Could you check a few things on this drawing? It's one solid part, dimensions in mm from its lowest x, y, z. A direction names the side the tool comes from. Give positions to 0.01 mm unless a question says otherwise; leave off trailing zeros. Write each loop counter-clockwise with the first axis right and the second up, starting at its lowest first coordinate (ties: lowest second). Pieces come first, ordered by that corner, then holes. Notation, with made-up numbers: M -14,18.25 L -10,18.25 A33 cw -10,51.25 Z; hole C 51,-26.5 d2. An arc over 180 degrees is marked long. Answer as CSV lines item,"result". Start each with the question number.
Q1. Suppose I cut it at B-B (y = 7.5). Write out the boundary of the cut face in (x, z), then the cut area to 3 significant figures.
Q2. Suppose I cut it at A-A (x = 23.5). Write out the boundary of the cut face in (y, z).
Q3. On a 3-axis mill with a long thin cutter (end or side, diameter ignored), from which of +Z, -Z, +X, -X, +Y, -Y can I reach the whole of each face in a straight line? I mean the marked faces 1 and 2. Say none if no direction works.
Q4. If I drill on line 1 along Y through (x, z) = (23.8, 37.5); line 2 along X through (y, z) = (5, 83); line 3 along Y through (x, z) = (16.25, 58.5), over which ranges is the centre line in solid material (lowest first)?
Q5. Suppose I cut it at C-C (z = 37.5). Write out the boundary of the cut face in (x, y).
Q6. Suppose I cut it at D-D (z = 55.5). Write out the boundary of the cut face in (x, y), then the cut area to 3 significant figures.
Q7. For pin 1 (2 mm diameter, centred on x = 8.5, z = 69.5, fed in from +Y); pin 2 (3 mm diameter, centred on y = 9, z = 34, fed in from -X), each with a flat end and sliding along its axis, tell me the tip position at first contact or that it passes through.
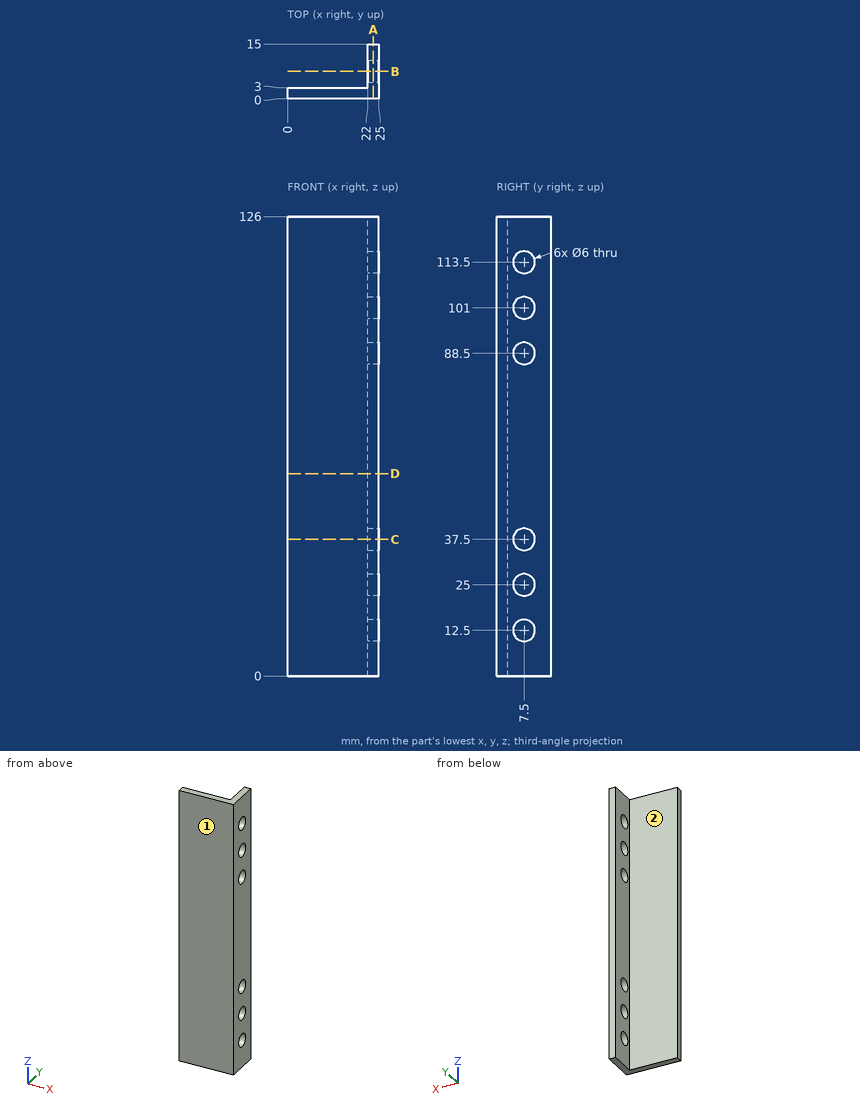
Resolved:
1,outline,"M 22,0 L 25,0 L 25,9.5 L 22,9.5 Z; M 22,15.5 L 25,15.5 L 25,22 L 22,22 Z; M 22,28 L 25,28 L 25,34.5 L 22,34.5 Z; M 22,40.5 L 25,40.5 L 25,85.5 L 22,85.5 Z; M 22,91.5 L 25,91.5 L 25,98 L 22,98 Z; M 22,104 L 25,104 L 25,110.5 L 22,110.5 Z; M 22,116.5 L 25,116.5 L 25,126 L 22,126 Z"
1,area,"270 mm^2"
2,outline,"M 0,0 L 15,0 L 15,126 L 0,126 Z; hole C 7.5,12.5 d6; hole C 7.5,25 d6; hole C 7.5,37.5 d6; hole C 7.5,88.5 d6; hole C 7.5,101 d6; hole C 7.5,113.5 d6"
3,face 1,"+Z, -Z, +X, -X, -Y"
3,face 2,"+Z, -Z, -X, +Y"
4,line 1,"0 to 4.5, 10.5 to 15"
4,line 2,"22 to 25"
4,line 3,"0 to 3"
5,outline,"M 0,0 L 25,0 L 25,4.5 L 22,4.5 L 22,3 L 0,3 Z; M 22,10.5 L 25,10.5 L 25,15 L 22,15 Z"
6,outline,"M 0,0 L 25,0 L 25,15 L 22,15 L 22,3 L 0,3 Z"
6,area,"111 mm^2"
7,pin 1,"y = 3"
7,pin 2,"x = 22"
